Autodesk Inventor part; units mm, degrees
ref_plane "YZ Plane" through (0, 0, 0) normal (1, 0, 0) x (0, 1, 0)
ref_plane "XZ Plane" through (0, 0, 0) normal (0, 1, 0) x (-1, 0, 0)
ref_plane "XY Plane" through (0, 0, 0) normal (0, 0, 1) x (1, 0, 0)
sketch "Szkic1" plane through (0, 0, 0) normal (0, 1, 0) x (-1, 0, 0)
  line L0 (-3.1297, -7.0475) -> (-3.1297, 9.5525)
  line L1 (17.6103, -7.0475) -> (-3.1297, -7.0475)
  line L2 (17.6103, 9.5525) -> (17.6103, -7.0475)
  line L3 (-3.1297, 9.5525) -> (17.6103, 9.5525)
  circle A0 centre (24.5703, 18.7775) radius 1.3
  circle A1 centre (-10.1297, -16.4225) radius 0.8
  line L4 (21.3203, -19.7725) -> (4.5808, -19.7725)
  line L5 (-16.2297, -14.5725) -> (-16.2297, 17.2275)
  line L6 (-13.2297, 20.2275) -> (28.0203, 20.2275)
  line L7 (32.0203, 16.2275) -> (32.0203, -13.0725)
  circle A2 centre (24.5703, 18.7775) radius 1.25
  line L8 (32.0203, 16.2275) -> (28.0203, 20.2275)
  arc A3 (-13.2297, 20.2275) -> (-16.2297, 17.2275) centre (-13.2297, 17.2275) ccw
  line L9 (4.5808, -19.7725) -> (0.7703, -17.5725)
  line L10 (0.7703, -17.5725) -> (-13.2297, -17.5725)
  line L11 (-13.2297, -17.5725) -> (-16.2297, -14.5725)
  line L12 (21.3203, -19.7725) -> (23.5203, -17.5725)
  line L13 (23.5203, -17.5725) -> (27.5203, -17.5725)
  line L14 (27.5203, -17.5725) -> (32.0203, -13.0725)
  line L15 (-13.1297, 17.1275) -> (27.6003, 17.1275)
  line L16 (27.6003, 17.1275) -> (27.6003, -14.6925)
  line L17 (27.6003, -14.6925) -> (-13.1297, -14.6925)
  line L18 (-13.1297, -14.6925) -> (-13.1297, 17.1275)
  circle A4 centre (28.5703, 17.4775) radius 1.25
  circle A5 centre (-14.5797, -14.5225) radius 1.25
  point P0 (0, 0)
  point P1 (-27.8297, -19.2225)
  point P2 (-15.1874, -15.6149)
  point P3 (-15.6721, -15.1301)
  point P4 (27.6003, 16.6891)
  point P5 (27.3703, 17.1275)
  dimension "d0" = 48.25
  dimension "d1" = 2.5
  dimension "d2" = 1.45
  dimension "d3" = 4
  dimension "d4" = 4
  dimension "d5" = 3
  dimension "d6" = 40
  dimension "d7" = 30
  dimension "d8" = 3
  dimension "d9" = 3
  dimension "d10" = 4.5
  dimension "d11" = 4.5
  dimension "d12" = 17
  dimension "d13" = 2.2
  dimension "d14" = 45
  dimension "d15" = 10.7
  dimension "d16" = 3.1
  dimension "d17" = 3.1
  dimension "d18" = 40.73
  dimension "d19" = 31.82
  dimension "d20" = 11.6
  dimension "d27" = 2.75
  dimension "d28" = 3.45
  dimension "d29" = 1.65
  dimension "d30" = 3.05
  dimension "d31" = 2.5
  dimension "d32" = 2.5
extrude "Wyciągnięcie proste1" add sketch "Szkic1" along normal blind 4 contours A0 | A1 | L4 L9 L10 L11 A5 L5 A3 L6 L8 L7 L14 L13 L12 | L11 A5 | A2 | A4 L16 L15 picked at (-14.8001, -14.1216) picked at (29.019, 17.6576)
extrude "Wyciągnięcie proste2" add sketch "Szkic1" along normal blind 1 contours L15 A4 L16 L17 L18 | L15 L16 A4 picked at (27.5683, 16.8804)
extrude "Wyciągnięcie proste3" add sketch "Szkic1" against normal blind 4.8 contours A0 | A1 | A2
extrude "Wyciągnięcie proste4" add sketch "Szkic1" along normal blind 9 contours L11 A5 | A4 L16 L15 | L15 L16 A4 picked at (-14.8001, -14.1216)
properties part number "podstawka"
Part model, mm, in its own coordinate system. A direction names the side the tool comes from. Give positions to 0.01 mm unless a question says otherwise; leave off trailing zeros. Order: outer loops, then holes, each group sorted by start corner. A loop starts at its lowest first (then second) coordinate and runs counter-clockwise, first axis right, second up. Notation, with made-up numbers: (-13.5, -31.5) - (30.5, -31.5) arc R17 ccw to (30.5, -22.5) - close; hole circle Ø4 at (-11, 45). An arc over 180 degrees is marked (long way). Use a Markdown table: item, result.
1) Probe L1, parallel to X at y = 6, z = 17.5; L2, parallel to Y at x = -23, z = -9; L3, parallel to Y at x = 5, z = -17. List the from-to ranges inside material, lowest first. Write a range as from..to.
Checked values:
| item | result |
|---|---|
| L1 | -29.82..-27.32 |
| L2 | 0..1 |
| L3 | 0..4 |
2) Saw through at C-C on z = -10.5. List the corners of the cut face in (x, y).
Checked values:
| item | result |
|---|---|
| outline | (-32.02, 0) - (16.23, 0) - (16.23, 4) - (13.13, 4) - (13.13, 1) - (-27.6, 1) - (-27.6, 4) - (-32.02, 4) - close |
3) Saw through at D-D on x = 8. List the corners of the cut face in (y, z).
Checked values:
| item | result |
|---|---|
| outline | (0, -17.57) - (4, -17.57) - (4, -14.69) - (1, -14.69) - (1, 17.13) - (4, 17.13) - (4, 20.23) - (0, 20.23) - close |
4) Flat gauge pins, fed straight in: P1, Ø6, axis at x = 3.5, z = 3.5, coming from the -Y side; P2, Ø20, axis at x = -15, z = 4, coming from the +Y side; P3, Ø2, axis at x = -2.5, y = 2.5, coming from the -Z side; P4, Ø1, axis at y = -2, z = -0.5, coming from the +X side. Where does each tip first touch, or does it go through?
Checked values:
| item | result |
|---|---|
| P1 | y = 0 |
| P2 | y = 1 |
| P3 | z = -19.15 |
| P4 | through |
5) 3-axis set-ups, long thin cutter, end or side, ignore diameter. For faces 1 (the flat face through (6, 2, -17.572)), 2 (the flat face through (-25, 2, -17.572)), 3 (the flat face through (-27.6, 2, 1)): which of +Z, -Z, +X, -X, +Y, -Y reach the whole face in a straight line?
Checked values:
| item | result |
|---|---|
| face 1 | -Z, +X, +Y, -Y |
| face 2 | -Z, -X, +Y, -Y |
| face 3 | +Y |
6) Saw through at A-A on z = 2. List the corners of the cut face in (x, y), plus the area to 3 significant figures.
Checked values:
| item | result |
|---|---|
| outline | (-32.02, 0) - (-17.61, 0) - (-17.61, 1) - (-27.6, 1) - (-27.6, 4) - (-32.02, 4) - close; (3.13, 0) - (16.23, 0) - (16.23, 4) - (13.13, 4) - (13.13, 1) - (3.13, 1) - close |
| area | 50.1 mm² |
7) Two-plate mould, pull along X, no slides. Class faces 4 (the flat face through (-7, 2, 17.128)), 5 (the cylindrical face through (9.76, -2.37, -17.13)), 6 (the flat face through (-29.74, 1.97, -15.35)): +X half, -X half, draft (parallel to the pull), parting line (faces both ways), or undercut.
Checked values:
| item | result |
|---|---|
| face 4 | undercut |
| face 5 | parting line |
| face 6 | -X half |
8) Saw through at B-B on x = -10. List the corners of the cut face in (y, z), plus the area to 3 significant figures.
Checked values:
| item | result |
|---|---|
| outline | (0, -19.77) - (4, -19.77) - (4, -14.69) - (1, -14.69) - (1, -7.05) - (0, -7.05) - close; (0, 9.55) - (1, 9.55) - (1, 17.13) - (4, 17.13) - (4, 20.23) - (0, 20.23) - close |
| area | 47.9 mm² |
